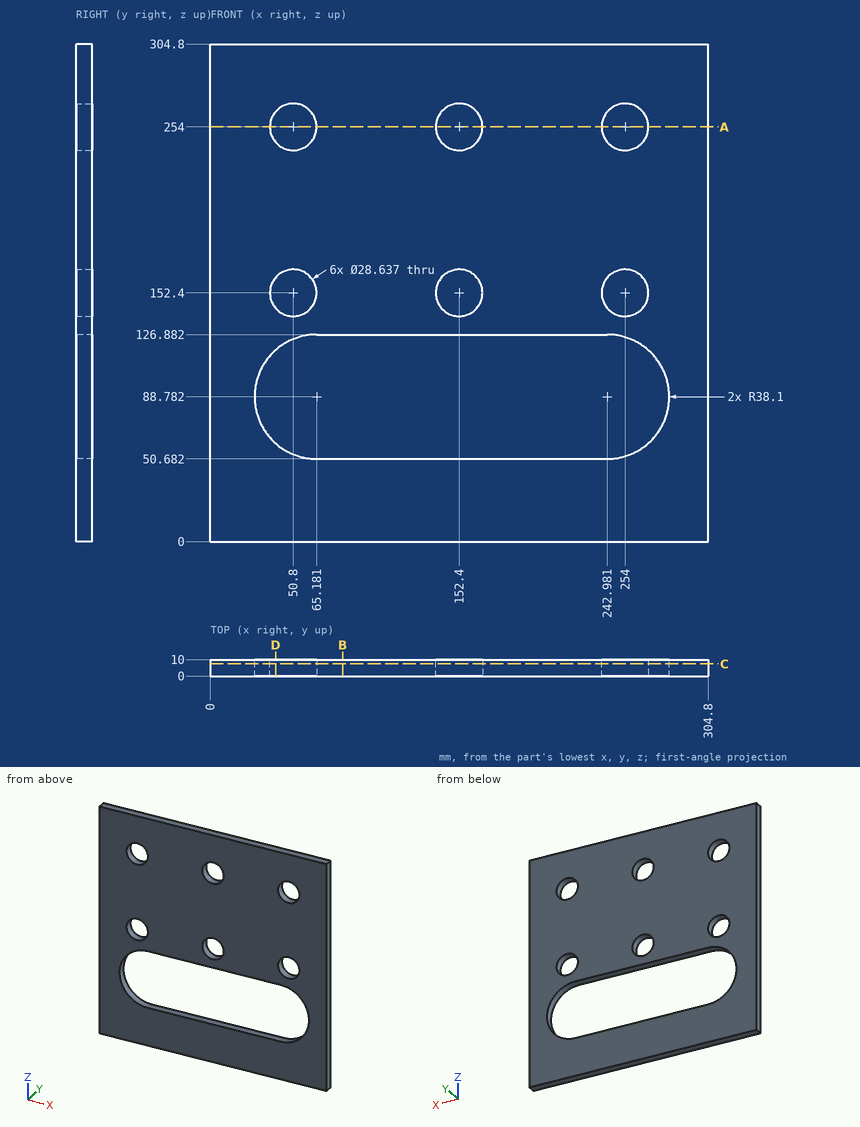
Drawing for the job (mm, zero at the part's lowest x, y, z). Give positions to 0.01 mm unless a question says otherwise; leave off trailing zeros. Order: outer loops, then holes, each group sorted by start corner. A loop starts at its lowest first (then second) coordinate and runs counter-clockwise, first axis right, second up. Notation, with made-up numbers: M 53.25,33.25 L 82.25,33.25 A23 ccw 82.25,54.25 Z; hole C -31,-28.5 d5. An arc over 180 degrees is marked long. Use a Markdown table: item, result. Add a question column.
(1) Saw through at D-D, the plane x = 40. Give the cut face in (y, z) (1 decimal).
(2) Drop a flat-ended pin along its axis: P1, Ø10, axis at x = 32, z = 95.5, coming from the +Y side. Give the stop position or say it passes through.
(3) Probe line 1 along Z through (x, y) = (152.4, 5.25); line 2 along X through (y, z) = (6, 161.5) (1 decimal); line 3 along Z through (x, y) = (130, 3.25). List the from-to ranges inside material, lowest first. Write a range as [from, to].
(4) Saw through at C-C, the plane y = 7.5. Give the cut face in (x, z), and give its area (3 significant figures).
(5) Saw through at B-B, the plane x = 81. Give the cut face in (y, z).
(6) Saw through at A-A, the plane z = 254. Give the cut face in (x, y).
Answer key:
| question | item | result |
|---|---|---|
| 1 | outline | M 0,0 L 10,0 L 10,60.2 L 0,60.2 Z; M 0,117.4 L 10,117.4 L 10,143 L 0,143 Z; M 0,161.8 L 10,161.8 L 10,244.6 L 0,244.6 Z; M 0,263.4 L 10,263.4 L 10,304.8 L 0,304.8 Z |
| 2 | P1 | y = 10 |
| 3 | line 1 | [0, 50.68], [126.88, 138.08], [166.72, 239.68], [268.32, 304.8] |
| 3 | line 2 | [0, 39.7], [61.9, 141.3], [163.5, 242.9], [265.1, 304.8] |
| 3 | line 3 | [0, 50.68], [126.88, 304.8] |
| 4 | outline | M 0,0 L 304.8,0 L 304.8,304.8 L 0,304.8 Z; hole C 50.8,152.4 d28.64; hole C 50.8,254 d28.64; hole M 65.18,50.68 L 242.98,50.68 A38.1 ccw 242.98,126.88 L 65.18,126.88 A38.1 ccw Z; hole C 152.4,152.4 d28.64; hole C 152.4,254 d28.64; hole C 254,152.4 d28.64; hole C 254,254 d28.64 |
| 4 | area | 70,900 mm^2 |
| 5 | outline | M 0,0 L 10,0 L 10,50.68 L 0,50.68 Z; M 0,126.88 L 10,126.88 L 10,304.8 L 0,304.8 Z |
| 6 | outline | M 0,0 L 36.48,0 L 36.48,10 L 0,10 Z; M 65.12,0 L 138.08,0 L 138.08,10 L 65.12,10 Z; M 166.72,0 L 239.68,0 L 239.68,10 L 166.72,10 Z; M 268.32,0 L 304.8,0 L 304.8,10 L 268.32,10 Z |
